Work out the finished part from the listing and answer in its coordinate system (mm). A direction names the side the tool comes from. Give positions to 0.01 mm unless a question says otherwise; leave off trailing zeros. Order: outer loops, then holes, each group sorted by start corner. A loop starts at its lowest first (then second) coordinate and runs counter-clockwise, first axis right, second up. Notation, with made-up numbers: (84, 33) - (102, 33) arc R26 ccw to (102, 60) - close; hole circle Ø2 at (1.5, 33.25). An arc over 180 degrees is marked (long way). Put each result on its own line as item: value.
```python
from build123d import *

# Parameters (mm, degrees)
F0_W     = 68.79
F0_H     = 25.61
F1_DEPTH = 25.61
F2_DEPTH = 100
F3_W     = 8.59875
F3_H     = 7.850625
F4_DEPTH = 50
F5_DEPTH = 51.308


with BuildPart() as f1:
    # F0 (on Top) → F1 (new body)
    with BuildSketch(Plane.XY):
        Rectangle(F0_W, F0_H)
    extrude(amount=F1_DEPTH)

    # F2 (add): a face of the model
    f2_faces = [f1.faces().sort_by_distance(p)[0] for p in [
        (0, 0, 0),
    ]]
    extrude(f2_faces, amount=F2_DEPTH)

    # F3 (on face) → F4 (cut)
    with BuildSketch(Plane.XZ.offset(12.805)):
        with Locations((-30.095625, -41.1203125)):
            Rectangle(F3_W, F3_H)
        with Locations((30.095625, -48.9709375)):
            Rectangle(F3_W, F3_H)
        with Locations((-30.095625, -56.8215625)):
            Rectangle(F3_W, F3_H)
        with Locations((30.095625, -64.6721875)):
            Rectangle(F3_W, F3_H)
        with Locations((-30.095625, -72.5228125)):
            Rectangle(F3_W, F3_H)
        with Locations((30.095625, -80.3734375)):
            Rectangle(F3_W, F3_H)
        with Locations((-30.095625, -88.2240625)):
            Rectangle(F3_W, F3_H)
    extrude(amount=-F4_DEPTH, mode=Mode.SUBTRACT)

    # F5 (cut): a face of the model
    f5_faces = [f1.faces().sort_by_distance(p)[0] for p in [
        (0, 0, 25.61),
    ]]
    extrude(f5_faces, amount=-F5_DEPTH, mode=Mode.SUBTRACT)


solid = f1.part
```
(1) Section B-B, the plane z = -55.5 is taken. Write down the section's boundary in (x, y) (3 decimals).
Geometry check:
outline: (-25.796, -12.805) - (34.395, -12.805) - (34.395, 12.805) - (-25.796, 12.805) - close
(2) Straight lines are drawn through the part: line 1 (Z direction, x = 29, y = 0); line 2 (Z direction, x = -30, y = -7.75) (1 decimal); line 3 (X direction, y = 9, z = -91) (3 decimals). For each, find the intervals that lie inside material, in ascending order.
Geometry check:
line 1: z = -100 to -84.3, -76.45 to -68.6, -60.75 to -52.9, -45.05 to -25.7
line 2: z = -100 to -92.1, -84.3 to -76.4, -68.6 to -60.7, -52.9 to -45, -37.2 to -25.7
line 3: x = -25.796 to 34.395
(3) Given pin 1 (1 mm diameter, centred on y = -7.5, z = -87, fed in from -X); pin 2 (4 mm diameter, centred on y = -1, z = -48, fed in from +X), each flat-ended and moving along its own axis, determine where each tip first touches the part or whether it passes through.
Geometry check:
pin 1: stops at x = -25.8
pin 2: stops at x = 25.8
(4) A tool of negligible diameter and unlimited length cuts with its end or side. For faces 4 (the face through (25.796, 0, -49)), 5 (the face through (-25.796, 0, -88)), 6 (the face through (0, 0, -25.698)), from which of +Z, -Z, +X, -X, +Y, -Y can it reach the whole face along a straight path? Write none if from no direction.
Geometry check:
face 4: +X, +Y, -Y
face 5: -X, +Y, -Y
face 6: +Z, +X, -X, +Y, -Y
(5) Determine the mould class of faces 1 (the face through (34.395, 0, -57)), 2 (the face through (-30, 0, -68.598)), 3 (the face through (0, 0, -100)) for opening direction Z: pulls with the +Z half, pulls with the -Z half, needs draft (parallel to the pull), parting line crosses it, or undercut.
Geometry check:
face 1: needs draft
face 2: undercut
face 3: pulls with the -Z half
